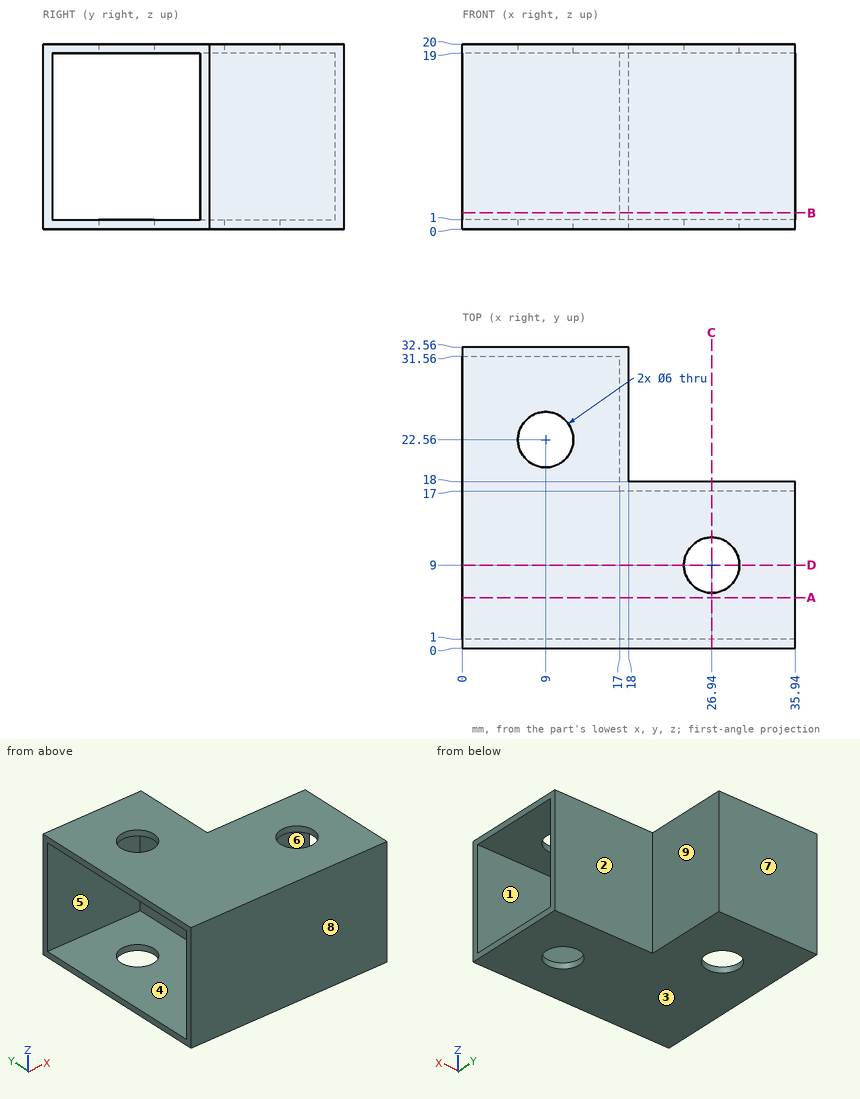
The drawing under review shows one solid part. Ordinate dimensions are in mm from its lowest x, y, z. A direction names the side the tool comes from. Round coordinates to 2 decimals unless told otherwise and drop trailing zeros. Write each loop counter-clockwise with the first axis right and the second up, starting at its lowest first coordinate (ties: lowest second). Pieces come first, ordered by that corner, then holes. Notation, with made-up numbers: (50, 38) - (97, 38) arc R18 cw to (97, 48) - close; hole circle Ø2 at (-33.75, 82). An arc over 180 degrees is marked (long way). Use a Markdown table: item, result. Add a question column.
1. Clearance check with flat-ended pins moving along their axes: pin 1 (5 mm diameter, centred on x = 26.94, y = 9, fed in from +Z); pin 2 (11.5 mm diameter, centred on y = 25.5, z = 12, fed in from +X); pin 3 (6 mm diameter, centred on y = 23.5, z = 9, fed in from -X); pin 4 (9 mm diameter, centred on x = 27.5, z = 12, fed in from +Y). State where each tip first meets the part, or that it passes through.
2. We need section B-B (z = 1.75). State the section outline as (x, y) points.
3. We need section D-D (y = 9). State the section outline as (x, z) points, then the cut area to 3 significant figures.
4. We need section C-C (x = 26.94). State the section outline as (y, z) points, then the cut area to 3 significant figures.
5. Mouldability with a two-part tool opening along Y and no side actions: class the marked faces 1, 2, 3 and 4 as +Y half, -Y half, draft (parallel to the pull), parting line (faces both ways), or undercut.
6. Wall thickness on probe 1 along Z at (x, y) = (32, 11); probe 2 along Y at (x, z) = (19, 6.5); probe 3 along Y at (x, z) = (9, 19.35): over which ranges is each line inside the solid? List them lowest first.
7. For the marked faces 5, 6, 7, 8 and 9, list the 3-axis set-ups (+Z, -Z, +X, -X, +Y, -Y) from which the entire face can be reached by the end or side of a thin tool; tool diameter is ignored.
8. We need section A-A (y = 5.5). State the section outline as (x, z) points.
Output:
| question | item | result |
|---|---|---|
| 1 | pin 1 | passes through |
| 1 | pin 2 | stops at x = 18 |
| 1 | pin 3 | stops at x = 17 |
| 1 | pin 4 | stops at y = 18 |
| 2 | outline | (0, 0) - (35.94, 0) - (35.94, 1) - (0, 1) - close; (0, 31.56) - (17, 31.56) - (17, 17) - (35.94, 17) - (35.94, 18) - (18, 18) - (18, 32.56) - (0, 32.56) - close |
| 3 | outline | (0, 0) - (23.94, 0) - (23.94, 1) - (0, 1) - close; (0, 19) - (23.94, 19) - (23.94, 20) - (0, 20) - close; (29.94, 0) - (35.94, 0) - (35.94, 1) - (29.94, 1) - close; (29.94, 19) - (35.94, 19) - (35.94, 20) - (29.94, 20) - close |
| 3 | area | 59.9 mm2 |
| 4 | outline | (0, 0) - (6, 0) - (6, 1) - (1, 1) - (1, 19) - (6, 19) - (6, 20) - (0, 20) - close; (12, 0) - (18, 0) - (18, 20) - (12, 20) - (12, 19) - (17, 19) - (17, 1) - (12, 1) - close |
| 4 | area | 60.0 mm2 |
| 5 | face 1 | undercut |
| 5 | face 2 | +Y half |
| 5 | face 3 | draft |
| 5 | face 4 | undercut |
| 6 | probe 1 | z = 0 to 1, 19 to 20 |
| 6 | probe 2 | y = 0 to 1, 17 to 18 |
| 6 | probe 3 | y = 0 to 19.56, 25.56 to 32.56 |
| 7 | face 5 | -X |
| 7 | face 6 | +X, -X |
| 7 | face 7 | +Z, -Z, +X, -X, +Y |
| 7 | face 8 | +Z, -Z, +X, -X, -Y |
| 7 | face 9 | +Z, -Z, +X, +Y |
| 8 | outline | (0, 0) - (35.94, 0) - (35.94, 1) - (0, 1) - close; (0, 19) - (35.94, 19) - (35.94, 20) - (0, 20) - close |
